Here's how the part is built. I have some questions about the finished solid (model axes, mm). Face numbers are marked on the shaded views. A direction names the side the tool comes from. Round coordinates to 2 decimals unless told otherwise and drop trailing zeros. Order: outer loops, then holes, each group sorted by start corner. A loop starts at its lowest first (then second) coordinate and runs counter-clockwise, first axis right, second up. Notation, with made-up numbers: (69.25, -31) -> (97.25, -31) arc R22 ccw to (97.25, -11) -> close; hole circle Ø2 at (-38.5, -28). An arc over 180 degrees is marked (long way). Use a Markdown table: item, result. Add a question column.
(1) On a 3-axis mill with a long thin cutter (end or side, diameter ignored), from which of +Z, -Z, +X, -X, +Y, -Y can I reach the whole of each face in a straight line? I mean the marked faces 5 and 6. Say none if no direction works.
(2) I want a section at D-D, the plane x = 3. Please give me the cut outline in (y, z), then the cut area to 3 significant figures.
(3) If I drill on probe 1 along Y at (x, z) = (-0.5, 2.5); probe 2 along Z at (x, y) = (-2.25, -3.5), over which ranges is the centre line in solid material (lowest first)?
(4) Thinking about a two-plate mould opening in Y: for the marked faces 1, 2, 3 and 4, which applies, pulls with the +Y half, pulls with the -Y half, needs draft (parallel to the pull), parting line crosses it, or undercut?
(5) I want a section at A-A, the plane z = 7. Please give me the cut outline in (x, y).
(6) I'm going to push a flat-ended pin straight in: P1, Ø2.5, axis at x = -1, y = 0, coming from the -Z side. Where does the tip first touch, or does it pass through?
(7) I want a section at B-B, the plane y = 0. Please give me the cut outline in (x, z) (3 decimals), then the cut area to 3 significant figures.
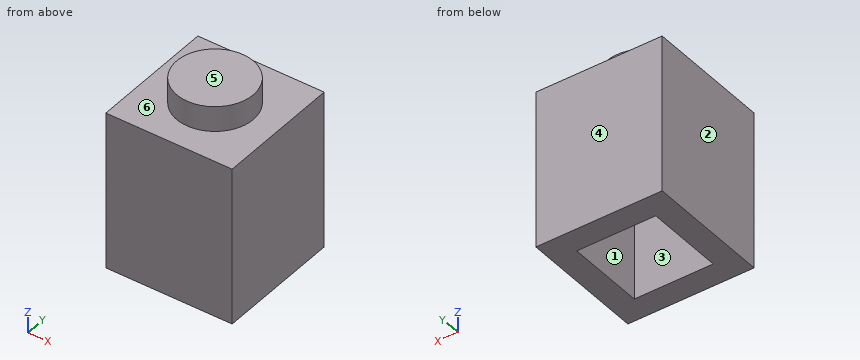
from build123d import *

# Parameters (mm, degrees)
F0_W     = 8
F0_H     = 8
F1_DEPTH = 10
F2_T     = -1.5
F3_R     = 2.425
F4_DEPTH = 1.6


with BuildPart() as f1:
    # F0 (on Top) → F1 (new body)
    with BuildSketch(Plane.XY):
        Rectangle(F0_W, F0_H)
    extrude(amount=F1_DEPTH)

    # F2
    f2_openings = [f1.faces().sort_by_distance(p)[0] for p in [
        (0, 0, 0),
    ]]
    offset(amount=F2_T, openings=f2_openings)

    # F3 (on face) → F4 (join)
    with BuildSketch(Plane.XY.offset(10)):
        Circle(F3_R)
    extrude(amount=F4_DEPTH)


solid = f1.part
Taken from the geometry:
| question | item | result |
|---|---|---|
| 1 | face 5 | +Z, +X, -X, +Y, -Y |
| 1 | face 6 | +Z |
| 2 | outline | (-4, 0) -> (4, 0) -> (4, 10) -> (-4, 10) -> close |
| 2 | area | 80.0 mm2 |
| 3 | probe 1 | y = -4 to -2.5, 2.5 to 4 |
| 3 | probe 2 | z = 0 to 10 |
| 4 | face 1 | undercut |
| 4 | face 2 | needs draft |
| 4 | face 3 | undercut |
| 4 | face 4 | pulls with the +Y half |
| 5 | outline | (-4, -4) -> (4, -4) -> (4, 4) -> (-4, 4) -> close; hole (-2.5, -2.5) -> (2.5, -2.5) -> (2.5, 2.5) -> (-2.5, 2.5) -> close |
| 6 | P1 | stops at z = 8.5 |
| 7 | outline | (-4, 0) -> (-2.5, 0) -> (-2.5, 8.5) -> (2.5, 8.5) -> (2.5, 0) -> (4, 0) -> (4, 10) -> (2.425, 10) -> (2.425, 11.6) -> (-2.425, 11.6) -> (-2.425, 10) -> (-4, 10) -> close |
| 7 | area | 45.3 mm2 |
